Work out the finished part from the listing and answer in its coordinate system (mm). A direction names the side the tool comes from. Round coordinates to 2 decimals unless told otherwise and drop trailing zeros. Order: outer loops, then holes, each group sorted by start corner. A loop starts at its lowest first (then second) coordinate and runs counter-clockwise, first axis right, second up.
from build123d import *

# Parameters (mm, degrees)
F0_W     = 13.288778
F0_H     = 6
F1_DEPTH = 25.4
F2_R     = 2
F3_DEPTH = 25.4
F4_R     = 2.462138
F5_DEPTH = 6.858


with BuildPart() as f1:
    # F0 (on Front) → F1 (new body)
    with BuildSketch(Plane.XZ):
        with Locations((-26.140303, 27.751791)):
            Rectangle(F0_W, F0_H)
    extrude(amount=F1_DEPTH)

    # F2 (on face) → F3 (cut)
    with BuildSketch(Plane.XY.offset(30.751791)):
        with Locations((-26.014924, -6.260172)):
            Circle(F2_R)
    extrude(amount=-F3_DEPTH, mode=Mode.SUBTRACT)

    # F4 (on face) → F5 (join)
    with BuildSketch(Plane.XY.offset(30.751791)):
        with Locations((-26.519462, -15.987486)):
            Circle(F4_R)
    extrude(amount=F5_DEPTH)


solid = f1.part
Item 1: Find section A-A (x = -25.75). Write down the section's boundary in (y, z).
Item 2: Find section B-B (y = -17.25). Write down the section's boundary in (x, z).
Item 3: Find the intervals of material crossed by line 1 along Z through (x, y) = (-29.5, -5.25); line 2 along Y through (x, z) = (-26.75, 27.25); line 3 along Y through (x, z) = (-27.25, 29.75), in increasing order.
Item 4: Given pin 1 (1.5 mm diameter, centred on x = -29.5, z = 35, fed in from -Y); pin 2 (3 mm diameter, centred on x = -30.5, y = -7.5, fed in from +Z); pin 3 (3 mm diameter, centred on x = -26.01, y = -6.26, fed in from +Z), each flat-ended and moving along its own axis, determine where each tip first touches the part or whether it passes through.
Item 5: A tool of negligible diameter and unlimited length cuts with its end or side. For faces 1 (the face through (-28.47, -17.49, 34.13)), 2 (the face through (-26, -13, 24.752)), from which of +Z, -Z, +X, -X, +Y, -Y can it reach the whole face along a straight path? Write none if from no direction.
Item 6: Find section D-D (x = -30.25). Write down the section's boundary in (y, z).
Item 7: Find section C-C (z = 28.75). Write down the section's boundary in (x, y).
Model answer:
1. outline: (-25.4, 24.75) - (-8.24, 24.75) - (-8.24, 30.75) - (-13.65, 30.75) - (-13.65, 37.61) - (-18.33, 37.61) - (-18.33, 30.75) - (-25.4, 30.75) - close; (-4.28, 24.75) - (0, 24.75) - (0, 30.75) - (-4.28, 30.75) - close
2. outline: (-32.78, 24.75) - (-19.5, 24.75) - (-19.5, 30.75) - (-24.41, 30.75) - (-24.41, 37.61) - (-28.63, 37.61) - (-28.63, 30.75) - (-32.78, 30.75) - close
3. line 1: z = 24.75 to 30.75
3. line 2: y = -25.4 to -8.12, -4.4 to 0
3. line 3: y = -25.4 to -7.83, -4.69 to 0
4. pin 1: stops at y = -17.03
4. pin 2: stops at z = 30.75
4. pin 3: passes through
5. face 1: +Z
5. face 2: -Z, +X, -X, +Y, -Y
6. outline: (-25.4, 24.75) - (0, 24.75) - (0, 30.75) - (-25.4, 30.75) - close
7. outline: (-32.78, -25.4) - (-19.5, -25.4) - (-19.5, 0) - (-32.78, 0) - close; hole circle Ø4 at (-26.01, -6.26)
